Can you work these out from the model? Positions are in its coordinate system, mm. A direction names the side the tool comes from. Give positions to 0.01 mm unless a question says otherwise; leave off trailing zeros. Loops run counter-clockwise (first coordinate to the right, second up) from the corner with the lowest first, then second, coordinate; pieces in that order, holes last. Notation, with made-up numbers: (-26.5, 80.25) - (27.5, 80.25) arc R25 ccw to (27.5, 95.25) - close; hole circle Ø11 at (-1, 55.25). An arc over 180 degrees is marked (long way). Answer in a Markdown table with one row per item.
from build123d import *

# Parameters (mm, degrees)
SKETCH1_R           = 5.5
SKETCH1_R_2         = 2.55
SKETCH1_R_3         = 1.6
BOSS_EXTRUDE1_DEPTH = 3
SKETCH2_R           = 8.05
CUT_EXTRUDE1_DEPTH  = 2


with BuildPart() as part:
    # Sketch1 → Boss-Extrude1 (new body)
    with BuildSketch(Plane(origin=(0, 0, 0), x_dir=(1, 0, 0), z_dir=(0, 1, 0))):
        with BuildLine():
            Line((-37.861879503, 50.161879503), (-18.657716447, 69.366042559))
            ThreePointArc((-18.657716447, 69.366042559), (-15.186386614, 71.685510998), (-11.091673888, 72.5))
            Line((-11.091673888, 72.5), (11.091673888, 72.5))
            ThreePointArc((11.091673888, 72.5), (15.186386614, 71.685510998), (18.657716447, 69.366042559))
            Line((18.657716447, 69.366042559), (37.861879503, 50.161879503))
            ThreePointArc((37.861879503, 50.161879503), (39.444320587, 47.793589056), (40, 45))
            Line((40, 45), (40, 5))
            ThreePointArc((40, 5), (38.535533906, 1.464466094), (35, 0))
            Line((35, 0), (-35, 0))
            ThreePointArc((-35, 0), (-38.535533906, 1.464466094), (-40, 5))
            Line((-40, 5), (-40, 45))
            ThreePointArc((-40, 45), (-39.444320587, 47.793589056), (-37.861879503, 50.161879503))
        make_face()
        with Locations((0, 32.5)):
            Circle(SKETCH1_R, mode=Mode.SUBTRACT)
        with Locations((0, 65.83)):
            Circle(SKETCH1_R_2, mode=Mode.SUBTRACT)
        with Locations((0, 54.4)):
            Circle(SKETCH1_R_3, mode=Mode.SUBTRACT)
        with Locations((-33.33, 32.5)):
            Circle(SKETCH1_R_2, mode=Mode.SUBTRACT)
        with Locations((-21.9, 32.5)):
            Circle(SKETCH1_R_3, mode=Mode.SUBTRACT)
        with Locations((33.33, 32.5)):
            Circle(SKETCH1_R_2, mode=Mode.SUBTRACT)
        with Locations((21.9, 32.5)):
            Circle(SKETCH1_R_3, mode=Mode.SUBTRACT)
        with BuildLine():
            Line((-2.5, 7.6), (-2.5, 16.4))
            ThreePointArc((-2.5, 16.4), (0, 18.9), (2.5, 16.4))
            Line((2.5, 16.4), (2.5, 7.6))
            ThreePointArc((2.5, 7.6), (0, 5.1), (-2.5, 7.6))
        make_face(mode=Mode.SUBTRACT)
        with BuildLine():
            Line((7.5, 7.6), (7.5, 16.4))
            ThreePointArc((7.5, 16.4), (10, 18.9), (12.5, 16.4))
            Line((12.5, 16.4), (12.5, 7.6))
            ThreePointArc((12.5, 7.6), (10, 5.1), (7.5, 7.6))
        make_face(mode=Mode.SUBTRACT)
        with BuildLine():
            Line((17.5, 7.6), (17.5, 16.4))
            ThreePointArc((17.5, 16.4), (20, 18.9), (22.5, 16.4))
            Line((22.5, 16.4), (22.5, 7.6))
            ThreePointArc((22.5, 7.6), (20, 5.1), (17.5, 7.6))
        make_face(mode=Mode.SUBTRACT)
        with BuildLine():
            Line((27.5, 7.6), (27.5, 16.4))
            ThreePointArc((27.5, 16.4), (30, 18.9), (32.5, 16.4))
            Line((32.5, 16.4), (32.5, 7.6))
            ThreePointArc((32.5, 7.6), (30, 5.1), (27.5, 7.6))
        make_face(mode=Mode.SUBTRACT)
        with BuildLine():
            Line((-7.5, 7.6), (-7.5, 16.4))
            ThreePointArc((-7.5, 16.4), (-10, 18.9), (-12.5, 16.4))
            Line((-12.5, 16.4), (-12.5, 7.6))
            ThreePointArc((-12.5, 7.6), (-10, 5.1), (-7.5, 7.6))
        make_face(mode=Mode.SUBTRACT)
        with BuildLine():
            Line((-17.5, 7.6), (-17.5, 16.4))
            ThreePointArc((-17.5, 16.4), (-20, 18.9), (-22.5, 16.4))
            Line((-22.5, 16.4), (-22.5, 7.6))
            ThreePointArc((-22.5, 7.6), (-20, 5.1), (-17.5, 7.6))
        make_face(mode=Mode.SUBTRACT)
        with BuildLine():
            Line((-27.5, 7.6), (-27.5, 16.4))
            ThreePointArc((-27.5, 16.4), (-30, 18.9), (-32.5, 16.4))
            Line((-32.5, 16.4), (-32.5, 7.6))
            ThreePointArc((-32.5, 7.6), (-30, 5.1), (-27.5, 7.6))
        make_face(mode=Mode.SUBTRACT)
    extrude(amount=BOSS_EXTRUDE1_DEPTH)

    # Sketch2 → Cut-Extrude1 (cut)
    with BuildSketch(Plane(origin=(0, 3, 0), x_dir=(1, 0, 0), z_dir=(0, 1, 0))):
        with Locations((0, 32.5)):
            Circle(SKETCH2_R)
    extrude(amount=-CUT_EXTRUDE1_DEPTH, mode=Mode.SUBTRACT)


solid = part.part
Q1. For pin 1 (1.9 mm diameter, centred on x = 21.9, z = -32.5, fed in from +Y); pin 2 (3 mm diameter, centred on x = 2, z = -37, fed in from +Y), each with a flat end and sliding along its axis, tell me the tip position at first contact or that it passes through.
Checked values:
| item | result |
|---|---|
| pin 1 | passes through |
| pin 2 | stops at y = 1 |
Q2. On a 3-axis mill with a long thin cutter (end or side, diameter ignored), from which of +Z, -Z, +X, -X, +Y, -Y can I reach the whole of each face in a straight line? I mean faces 1 (the face through (-28.394, 1.479, -59.63)), 2 (the face through (-29.9, 1.5, -18.9)), 3 (the face through (2, 1, -27)). Say none if no direction works.
Checked values:
| item | result |
|---|---|
| face 1 | -Z, -X, +Y, -Y |
| face 2 | +Y, -Y |
| face 3 | +Y |
Q3. Imagine slicing it at B-B, the plane z = -32.5. Write out the boundary of the cut face in (x, y), and give its area (3 significant figures).
Checked values:
| item | result |
|---|---|
| outline | (-40, 0) - (-35.88, 0) - (-35.88, 3) - (-40, 3) - close; (-30.78, 0) - (-23.5, 0) - (-23.5, 3) - (-30.78, 3) - close; (-20.3, 0) - (-5.5, 0) - (-5.5, 1) - (-8.05, 1) - (-8.05, 3) - (-20.3, 3) - close; (5.5, 0) - (20.3, 0) - (20.3, 3) - (8.05, 3) - (8.05, 1) - (5.5, 1) - close; (23.5, 0) - (30.78, 0) - (30.78, 3) - (23.5, 3) - close; (35.88, 0) - (40, 0) - (40, 3) - (35.88, 3) - close |
| area | 147 mm² |
Q4. Imagine slicing it at A-A, the plane x = -10. Write out the boundary of the cut face in (y, z).
Checked values:
| item | result |
|---|---|
| outline | (0, -72.5) - (3, -72.5) - (3, -18.9) - (0, -18.9) - close; (0, -5.1) - (3, -5.1) - (3, 0) - (0, 0) - close |
Q5. Imagine slicing it at D-D, the plane z = -17.5. Count the separate pieces of the cut face and the enclosed holes in it, and give its area (3 significant figures).
Checked values:
| item | result |
|---|---|
| separate pieces | 8 |
| enclosed holes | 0 |
| area | 146 mm² |
Q6. If I drill on line 1 (X direction, y = 0.6, z = -32.5); line 2 (Z direction, x = 0, y = 0.65); line 3 (X direction, y = 2.15, z = -65.83), over which ranges is the centre line in solid material (lowest first)? Write a range as [from, to].
Checked values:
| item | result |
|---|---|
| line 1 | x = [-40, -35.88], [-30.78, -23.5], [-20.3, -5.5], [5.5, 20.3], [23.5, 30.78], [35.88, 40] |
| line 2 | z = [-72.5, -68.38], [-63.28, -56], [-52.8, -38], [-27, -18.9], [-5.1, 0] |
| line 3 | x = [-22.19, -2.55], [2.55, 22.19] |
Q7. Imagine slicing it at C-C, the plane x = 0. Write out the boundary of the cut face in (y, z).
Checked values:
| item | result |
|---|---|
| outline | (0, -72.5) - (3, -72.5) - (3, -68.38) - (0, -68.38) - close; (0, -63.28) - (3, -63.28) - (3, -56) - (0, -56) - close; (0, -52.8) - (3, -52.8) - (3, -40.55) - (1, -40.55) - (1, -38) - (0, -38) - close; (0, -27) - (1, -27) - (1, -24.45) - (3, -24.45) - (3, -18.9) - (0, -18.9) - close; (0, -5.1) - (3, -5.1) - (3, 0) - (0, 0) - close |
Q8. If we mould it in two halves opening along Z, with no side actions, what happens to faces 4 (the face through (-32.5, 1, -12)), 5 (the face through (0, 1, -72.5)), 6 (the face through (22.5, 1, -12))? For each: released by +Z, released by -Z, zero draft, split by the parting line, or undercut.
Checked values:
| item | result |
|---|---|
| face 4 | undercut |
| face 5 | released by -Z |
| face 6 | undercut |
